```python
from build123d import *

# Parameters (mm, degrees)
SZKIC1_W                    = 121
SZKIC1_H                    = 24
SZKIC1_R                    = 2.1
DODANIE_WYCI_GNI_CIE1_DEPTH = 5
SZKIC2_W                    = 18
SZKIC2_H                    = 21
DODANIE_WYCI_GNI_CIE2_DEPTH = 36
WYTNIJ_WYCI_GNI_CIE1_REACH  = 76.062
SZKIC3_R                    = 1.75
SZKIC4_R                    = 3.75
WYTNIJ_WYCI_GNI_CIE2_DEPTH  = 38
ZAOKR_GLENIE1_R             = 0.9
SZKIC5_W                    = 121
SZKIC5_H                    = 1.5
DODANIE_WYCI_GNI_CIE3_DEPTH = 45
SZKIC6_W                    = 18
SZKIC6_H                    = 36
WYTNIJ_WYCI_GNI_CIE3_DEPTH  = 0.2
SZKIC7_W                    = 18
SZKIC7_H                    = 4.2
WYTNIJ_WYCI_GNI_CIE4_DEPTH  = 1.4
SZKIC8_W                    = 2
SZKIC8_H                    = 20
SZKIC8_W_2                  = 1.5
DODANIE_WYCI_GNI_CIE4_DEPTH = 20.8
SFAZOWANIE1_SIZE            = 1
SFAZOWANIE2_SIZE            = 1


with BuildPart() as part:
    # Szkic1 → Dodanie-wyciągnięcie1 (new body)
    with BuildSketch(Plane.XY):
        Rectangle(SZKIC1_W, SZKIC1_H)
        with Locations((-40, 0)):
            Circle(SZKIC1_R, mode=Mode.SUBTRACT)
        with Locations((40, 0)):
            Circle(SZKIC1_R, mode=Mode.SUBTRACT)
    extrude(amount=DODANIE_WYCI_GNI_CIE1_DEPTH)

    # Szkic2 → Dodanie-wyciągnięcie2 (add)
    with BuildSketch(Plane.XY.offset(5)):
        Rectangle(SZKIC2_W, SZKIC2_H)
    extrude(amount=DODANIE_WYCI_GNI_CIE2_DEPTH)

    # Szkic3 → Wytnij-wyciągnięcie1 (cut, up to next)
    with BuildSketch(Plane.XY.offset(41), mode=Mode.PRIVATE) as wytnij_wyci_gni_cie1_sk1:
        with Locations((-5.5, 5.45)):
            Circle(SZKIC3_R)
    wytnij_wyci_gni_cie1_tool1 = extrude(wytnij_wyci_gni_cie1_sk1.sketch, amount=-WYTNIJ_WYCI_GNI_CIE1_REACH, mode=Mode.PRIVATE) & part.part
    # Szkic3 → Wytnij-wyciągnięcie1 (cut, up to next)
    with BuildSketch(Plane.XY.offset(41), mode=Mode.PRIVATE) as wytnij_wyci_gni_cie1_sk2:
        with Locations((-5.5, -5.45)):
            Circle(SZKIC3_R)
    wytnij_wyci_gni_cie1_tool2 = extrude(wytnij_wyci_gni_cie1_sk2.sketch, amount=-WYTNIJ_WYCI_GNI_CIE1_REACH, mode=Mode.PRIVATE) & part.part
    # Szkic3 → Wytnij-wyciągnięcie1 (cut, up to next)
    with BuildSketch(Plane.XY.offset(41), mode=Mode.PRIVATE) as wytnij_wyci_gni_cie1_sk3:
        with Locations((5.5, -5.45)):
            Circle(SZKIC3_R)
    wytnij_wyci_gni_cie1_tool3 = extrude(wytnij_wyci_gni_cie1_sk3.sketch, amount=-WYTNIJ_WYCI_GNI_CIE1_REACH, mode=Mode.PRIVATE) & part.part
    # Szkic3 → Wytnij-wyciągnięcie1 (cut, up to next)
    with BuildSketch(Plane.XY.offset(41), mode=Mode.PRIVATE) as wytnij_wyci_gni_cie1_sk4:
        with Locations((5.5, 5.45)):
            Circle(SZKIC3_R)
    wytnij_wyci_gni_cie1_tool4 = extrude(wytnij_wyci_gni_cie1_sk4.sketch, amount=-WYTNIJ_WYCI_GNI_CIE1_REACH, mode=Mode.PRIVATE) & part.part
    add(wytnij_wyci_gni_cie1_tool1.solids().sort_by_distance((-5.5, 5.45, 41))[0], mode=Mode.SUBTRACT)
    add(wytnij_wyci_gni_cie1_tool2.solids().sort_by_distance((-5.5, -5.45, 41))[0], mode=Mode.SUBTRACT)
    add(wytnij_wyci_gni_cie1_tool3.solids().sort_by_distance((5.5, -5.45, 41))[0], mode=Mode.SUBTRACT)
    add(wytnij_wyci_gni_cie1_tool4.solids().sort_by_distance((5.5, 5.45, 41))[0], mode=Mode.SUBTRACT)

    # Szkic4 → Wytnij-wyciągnięcie2 (cut)
    with BuildSketch(Plane(origin=(0, 0, 0), x_dir=(-1, 0, 0), z_dir=(0, 0, -1))):
        with Locations((-5.5, 5.45)):
            Circle(SZKIC4_R)
        with Locations((-5.5, -5.45)):
            Circle(SZKIC4_R)
        with Locations((5.5, 5.45)):
            Circle(SZKIC4_R)
        with Locations((5.5, -5.45)):
            Circle(SZKIC4_R)
    extrude(amount=-WYTNIJ_WYCI_GNI_CIE2_DEPTH, mode=Mode.SUBTRACT)

    # Zaokrąglenie1
    zaokr_glenie1_edges = [part.edges().sort_by_distance(p)[0] for p in [
        (-9, -4.103708798, 21.5),
        (-9, -6.796291202, 21.5),
        (-9, 6.796291202, 21.5),
        (-9, 4.103708798, 21.5),
        (9, 4.103708798, 21.5),
        (9, 6.796291202, 21.5),
        (9, -6.796291202, 21.5),
        (9, -4.103708798, 21.5),
    ]]
    fillet(zaokr_glenie1_edges, radius=ZAOKR_GLENIE1_R)

    # Szkic5 → Dodanie-wyciągnięcie3 (add)
    with BuildSketch(Plane.XY.offset(5)):
        with Locations((0, -11.25)):
            Rectangle(SZKIC5_W, SZKIC5_H)
    extrude(amount=DODANIE_WYCI_GNI_CIE3_DEPTH)

    # Szkic6 → Wytnij-wyciągnięcie3 (cut)
    with BuildSketch(Plane(origin=(0, 10.5, 0), x_dir=(1, 0, 0), z_dir=(0, 1, 0))):
        with Locations((0, -23)):
            Rectangle(SZKIC6_W, SZKIC6_H)
    extrude(amount=-WYTNIJ_WYCI_GNI_CIE3_DEPTH, mode=Mode.SUBTRACT)

    # Szkic7 → Wytnij-wyciągnięcie4 (cut)
    with BuildSketch(Plane(origin=(0, 10.3, 0), x_dir=(1, 0, 0), z_dir=(0, 1, 0))):
        with Locations((0, -7.1)):
            Rectangle(SZKIC7_W, SZKIC7_H)
    extrude(amount=-WYTNIJ_WYCI_GNI_CIE4_DEPTH, mode=Mode.SUBTRACT)

    # Szkic8 → Dodanie-wyciągnięcie4 (add)
    with BuildSketch(Plane(origin=(0, -10.5, 0), x_dir=(1, 0, 0), z_dir=(0, 1, 0))):
        with Locations((-59.5, -15)):
            Rectangle(SZKIC8_W, SZKIC8_H)
        with Locations((59.75, -15)):
            Rectangle(SZKIC8_W_2, SZKIC8_H)
    extrude(amount=DODANIE_WYCI_GNI_CIE4_DEPTH)

    # Sfazowanie1
    sfazowanie1_edges = [part.edges().sort_by_distance(p)[0] for p in [
        (0, -12, 0),
        (-60.5, 0, 0),
        (0, 12, 0),
        (60.5, 0, 0),
    ]]
    chamfer(sfazowanie1_edges, length=SFAZOWANIE1_SIZE)

    # Sfazowanie2
    sfazowanie2_edges = [part.edges().sort_by_distance(p)[0] for p in [
        (60.5, -12, 25.5),
        (-60.5, -12, 25.5),
        (-60.5, 12, 3),
        (60.5, 12, 3),
    ]]
    chamfer(sfazowanie2_edges, length=SFAZOWANIE2_SIZE)


solid = part.part
```
Geometry check sheet. Reference: the model listing, model coordinates, mm. A direction names the side the tool comes from. Round coordinates to 2 decimals unless told otherwise and drop trailing zeros. Order: outer loops, then holes, each group sorted by start corner. A loop starts at its lowest first (then second) coordinate and runs counter-clockwise, first axis right, second up. Notation, with made-up numbers: (69.5, 14.25) - (109.5, 14.25) arc R19 ccw to (109.5, 36.25) - close; hole circle Ø7 at (24.5, 46). An arc over 180 degrees is marked (long way). Use a Markdown table: item, result. Add a question column.
1) Section check C-C (y = 0). Record the cut outline in (x, z).
2) Thickness scan on line 1 along X through (y, z) = (5.45, 16); line 2 along X through (y, z) = (-5.75, 40); line 3 along Y through (x, z) = (-5.5, 32). Record the ranges inside material, lowest first.
3) Section check D-D (x = -40). Record the cut outline in (y, z).
4) Gauge pin test, flat ends, axial feed: P1, Ø5, axis at x = 39.5, z = 35, coming from the +Y side; P2, Ø1.5, axis at x = 0, z = 18.5, coming from the +Y side; P3, Ø4.5, axis at x = 5.5, y = 5.45, coming from the -Z side. Record the tip position at first contact, or that the pin passes through.
5) Section check A-A (y = -5.45). Count the separate pieces of the cut face and the enclosed holes in it, then the cut area to 4 significant figures.
6) Set-up check for faces 1 (the flat face through (9, -1, 26)), 2 (the flat face through (-60, 0, 25)), 3 (the cylindrical face through (-1.754, 5.615, 18.734)): record each of +Z, -Z, +X, -X, +Y, -Y from which the full face is reachable in a straight line by a thin tool's end or side.
7) Section check B-B (x = 5.5). Record the cut outline in (y, z).
8) Mould release check, pull along X, two halves, no side actions. Record for faces 4 (the cylindrical face through (4.1, 4.4, 39.5)), 5 (the flat face through (-60.5, 0, 15)), 6 (the flat face through (-1, -12, 25)): released by +X, released by -X, zero draft, split by the parting line, or undercut.
Established:
| question | item | result |
|---|---|---|
| 1 | outline | (-60.5, 1) - (-59.5, 0) - (-42.1, 0) - (-42.1, 5) - (-58.5, 5) - (-58.5, 25) - (-60.5, 25) - close; (-37.9, 0) - (37.9, 0) - (37.9, 5) - (9, 5) - (9, 41) - (-9, 41) - (-9, 5) - (-37.9, 5) - close; (42.1, 0) - (59.5, 0) - (60.5, 1) - (60.5, 25) - (59, 25) - (59, 5) - (42.1, 5) - close |
| 2 | line 1 | -60.5 to -58.5, -1.75 to 1.75, 59 to 60.5 |
| 2 | line 2 | -9 to -7.22, -3.78 to 3.78, 7.22 to 9 |
| 2 | line 3 | -12 to -9.2, -1.7 to 1.7, 9.2 to 10.3 |
| 3 | outline | (-12, 1) - (-11, 0) - (-2.1, 0) - (-2.1, 5) - (-10.5, 5) - (-10.5, 50) - (-12, 50) - close; (2.1, 0) - (11, 0) - (12, 1) - (12, 5) - (2.1, 5) - close |
| 4 | P1 | y = -10.5 |
| 4 | P2 | y = 10.3 |
| 4 | P3 | z = 38 |
| 5 | separate pieces | 5 |
| 5 | enclosed holes | 0 |
| 5 | area | 747.5 mm2 |
| 6 | face 1 | +Z, +Y |
| 6 | face 2 | +Z, -X, +Y |
| 6 | face 3 | -Z |
| 7 | outline | (-12, 1) - (-11, 0) - (-9.2, 0) - (-9.2, 38) - (-7.2, 38) - (-7.2, 41) - (-10.5, 41) - (-10.5, 50) - (-12, 50) - close; (-3.7, 38) - (-1.7, 38) - (-1.7, 0) - (1.7, 0) - (1.7, 38) - (3.7, 38) - (3.7, 41) - (-3.7, 41) - close; (7.2, 38) - (9.2, 38) - (9.2, 9.2) - (10.3, 9.2) - (10.3, 41) - (7.2, 41) - close; (9.2, 0) - (11, 0) - (12, 1) - (12, 5) - (9.2, 5) - close |
| 8 | face 4 | undercut |
| 8 | face 5 | released by -X |
| 8 | face 6 | zero draft |
